For this review, use the dimensioned drawing (mm, ordinates from the lowest corner) and the shaded views. A direction names the side the tool comes from. Coordinates: 2 decimals unless noted, no trailing zeros. Write each loop counter-clockwise with the first axis right and the second up, starting at its lowest first coordinate (ties: lowest second). Pieces come first, ordered by that corner, then holes. Notation, with made-up numbers: (-21, 26.5) - (19, 26.5) arc R32 cw to (19, 59.5) - close; hole circle Ø8 at (-4, -18.5). An arc over 180 degrees is marked (long way). Answer as a JSON object with one key per item and string values.
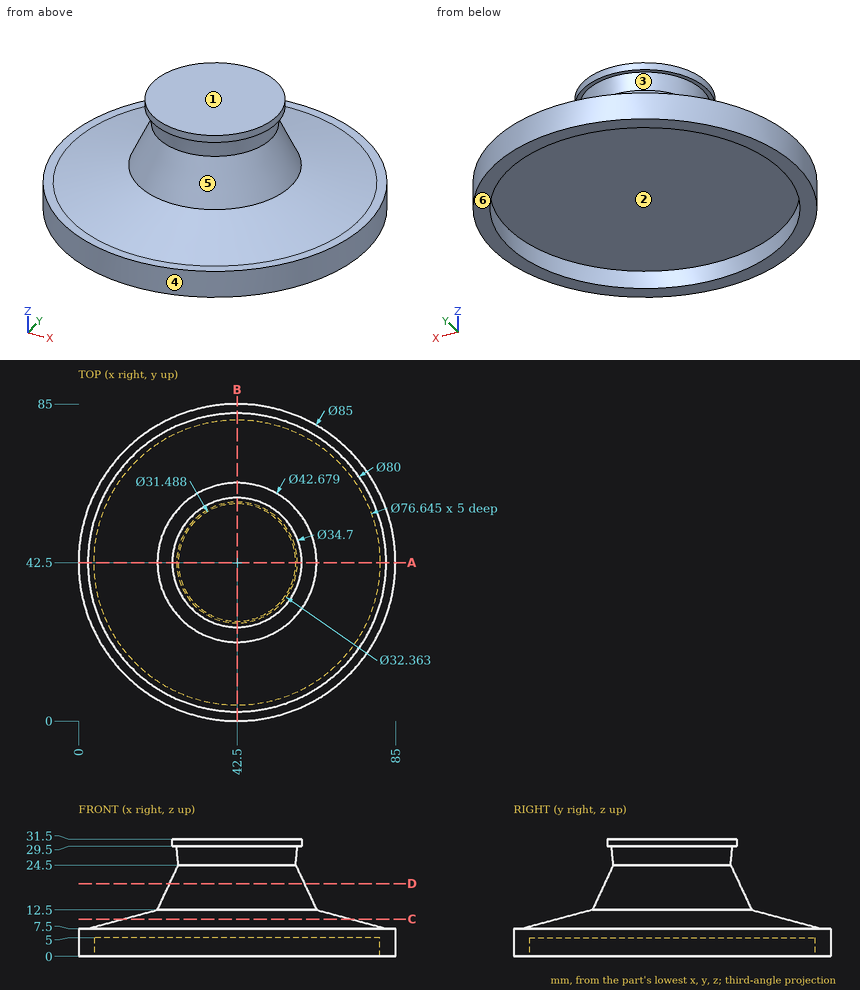
(1) To check wall thickness, follow line 1 (X direction, y = 42, z = 1); line 2 (X direction, y = 31, z = 2) (1 decimal). State the ranges of each line that lie inside material, in increasing order. Write a range as from..to.
Solved:
{"line 1": "x = 0..4.18, 80.82..85", "line 2": "x = 1.6..5.9, 79.1..83.4"}
(2) Take a section at A-A, the plane y = 42.5. Write out the cut boundary in (x, z).
Solved:
{"outline": "(0, 0) - (4.18, 0) - (4.18, 5) - (80.82, 5) - (80.82, 0) - (85, 0) - (85, 7.5) - (82.5, 7.5) - (63.84, 12.5) - (58.24, 24.5) - (58.68, 29.5) - (59.85, 29.5) - (59.85, 31.5) - (25.15, 31.5) - (25.15, 29.5) - (26.32, 29.5) - (26.76, 24.5) - (21.16, 12.5) - (2.5, 7.5) - (0, 7.5) - close"}
(3) For pin 1 (3 mm diameter, centred on x = 34.5, z = 6, fed in from -Y); pin 2 (8 mm diameter, centred on x = 42, z = 5, fed in from -Y); pin 3 (2 mm diameter, centred on x = 54, z = 27.5, fed in from +Y), all flat-tipped, find the tip position at first contact; note any pin that passes through.
Solved:
{"pin 1": "stops at y = 0.5", "pin 2": "stops at y = 0", "pin 3": "stops at y = 54.59"}
(4) Take a section at D-D, the plane z = 19.5. Write out the cut boundary in (x, y) (1 decimal), and give its area (3 significant figures).
Solved:
{"outline": "circle Ø36.2 at (42.5, 42.5)", "area": "1,030 mm^2"}
(5) Take a section at C-C, the plane z = 10. Write out the cut boundary in (x, y), and give its area (4 significant figures).
Solved:
{"outline": "circle Ø61.34 at (42.5, 42.5)", "area": "2,955 mm^2"}
(6) The part is to be moulded in two halves that separate along Z. For the marked faces 4, 5 and 6, say which applies: pulls with the +Z half, pulls with the -Z half, needs draft (parallel to the pull), parting line crosses it, or undercut.
Solved:
{"face 4": "needs draft", "face 5": "undercut", "face 6": "pulls with the -Z half"}
(7) Tool access review of the marked faces 1, 2 and 3: name each direction out of +Z, -Z, +X, -X, +Y, -Y from which nothing blocks a thin tool from reaching the whole face with its end or side.
Solved:
{"face 1": "+Z, +X, -X, +Y, -Y", "face 2": "-Z", "face 3": "none"}
